Geometry: see drawing. Coordinates: mm, zero at the bounding-box minimum. A direction names the side the tool comes from. Give positions to 0.01 mm unless a question says otherwise; leave off trailing zeros. Write each loop counter-clockwise with the first axis right and the second up, starting at its lowest first coordinate (ties: lowest second). Pieces come first, ordered by that corner, then holes. Notation, with made-up numbers: M 63.5,65.25 L 101.5,65.25 A22 ccw 101.5,79.25 Z; hole C 84,57 d11. An arc over 180 degrees is marked long. Use a Markdown table: item, result. Add a question column.
(1) Cut plane B-B (z = 10.5). Output: boundary loops of the cut face in (x, y) (3 decimals).
(2) Cut plane C-C (z = 5.5). Output: boundary loops of the cut face in (x, y) (3 decimals), plus the area to 3 significant figures.
(3) Cut plane D-D (x = 21). Output: boundary loops of the cut face in (y, z), plus the area to 3 significant figures.
(4) Material intervals for L1, parallel to X at y = 2.75, z = 8.5 (3 decimals); L2, parallel to X at y = 5.5, z = 12.5 (3 decimals); L3, parallel to Z at x = 22.5, y = 4.75, sorted ascending.
(5) Cut plane A-A (y = 4.5). Output: boundary loops of the cut face in (x, z) (3 decimals).
(6) Pin query (flat end, axial travel): pin 1 Ø3 at (x, y) = (19, 2) entering from +Z; pin 2 Ø1.9 at (y, z) = (4.5, 14) entering from -X; pin 3 Ø4 at (x, z) = (26, 6.5) entering from +Y. Return the tip coordinate at first contact, or that it passes through.
(7) Draft query along X for the marked faces 3, 4 and 5. Return one class per face: released by +X, released by -X, zero draft, split by the parting line, or undercut.
(8) Reachability of the marked faces 1 and 2 from +Z, -Z, +X, -X, +Y, -Y: full face, straight path, thin tool, end or side. Return the list, or none.
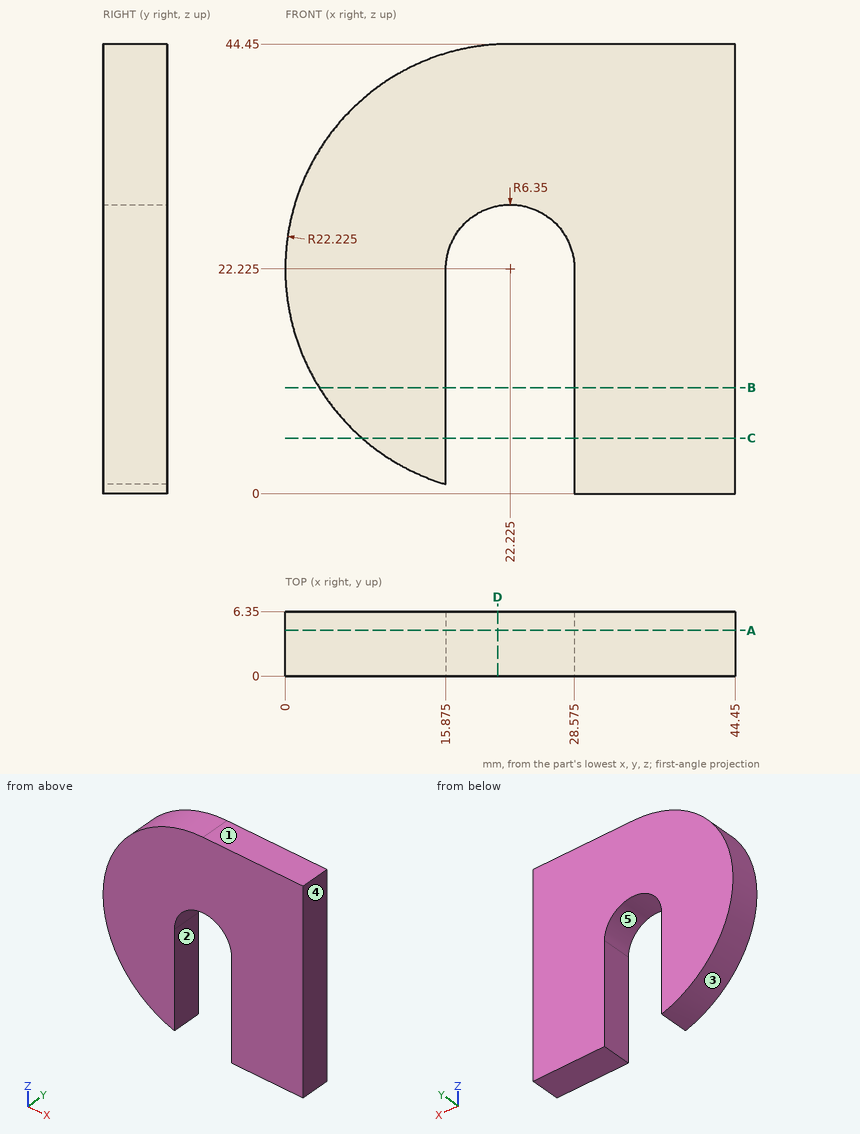
Answer list:
| question | item | result |
|---|---|---|
| 1 | outline | M 3.344,0 L 15.875,0 L 15.875,6.35 L 3.344,6.35 Z; M 28.575,0 L 44.45,0 L 44.45,6.35 L 28.575,6.35 Z |
| 2 | outline | M 7.589,0 L 15.875,0 L 15.875,6.35 L 7.589,6.35 Z; M 28.575,0 L 44.45,0 L 44.45,6.35 L 28.575,6.35 Z |
| 2 | area | 153 mm² |
| 3 | outline | M 0,28.46 L 6.35,28.46 L 6.35,44.42 L 0,44.42 Z |
| 3 | area | 101 mm² |
| 4 | L1 | 4.744 to 15.875, 28.575 to 44.45 |
| 4 | L2 | 2.241 to 15.875, 28.575 to 44.45 |
| 4 | L3 | 28.57 to 44.45 |
| 5 | outline | M 15.875,0.926 L 15.875,22.225 A6.35 cw 28.575,22.225 L 28.575,0 L 44.45,0 L 44.45,44.45 L 22.225,44.45 A22.225 ccw Z |
| 6 | pin 1 | z = 44.38 |
| 6 | pin 2 | x = 1.22 |
| 6 | pin 3 | through |
| 7 | face 3 | released by -X |
| 7 | face 4 | released by +X |
| 7 | face 5 | undercut |
| 8 | face 1 | +Z, +X, -X, +Y, -Y |
| 8 | face 2 | -Z, +Y, -Y |
